Here's how the part is built. I have some questions about the finished solid (model axes, mm). A direction names the side the tool comes from. Round coordinates to 2 decimals unless told otherwise and drop trailing zeros. Order: outer loops, then holes, each group sorted by start corner. A loop starts at its lowest first (then second) coordinate and runs counter-clockwise, first axis right, second up.
```python
from build123d import *

# Parameters (mm, degrees)
SKETCH1_R           = 14.2875
SKETCH1_R_2         = 7.9375
SKETCH1_R_3         = 3.429
SKETCH1_R_4         = 2.54
BOSS_EXTRUDE1_DEPTH = 6.35


with BuildPart() as part:
    # Sketch1 → Boss-Extrude1 (new body)
    with BuildSketch(Plane(origin=(0, 0, 0), x_dir=(0, 0, -1), z_dir=(1, 0, 0))):
        with BuildLine():
            Line((12.7, -88.9), (-1.575652176, -88.9))
            ThreePointArc((-1.575652176, -88.9), (-4.987504689, -87.905535681), (-7.330706623, -85.233625962))
            Line((-7.330706623, -85.233625962), (-16.304501832, -65.989260033))
            ThreePointArc((-16.304501832, -65.989260033), (-19.450268482, -62.883748133), (-23.860481018, -62.583619201))
            ThreePointArc((-23.860481018, -62.583619201), (-35.194449796, -57.475157953), (-31.822423449, -45.509178558))
            ThreePointArc((-31.822423449, -45.509178558), (-29.217505575, -41.937840594), (-29.574405884, -37.53185896))
            Line((-29.574405884, -37.53185896), (-42.070217791, -10.734503848))
            ThreePointArc((-42.070217791, -10.734503848), (-44.064116927, 4.410663713), (-37.010512242, 17.960512242))
            Line((-37.010512242, 17.960512242), (5.544864644, 60.515889128))
            ThreePointArc((5.544864644, 60.515889128), (12.382451565, 63.66408435), (19.411500847, 60.970351952))
            Line((19.411500847, 60.970351952), (75.796601185, 6.873195536))
            ThreePointArc((75.796601185, 6.873195536), (78.685483549, 0.891546289), (76.962077301, -5.523719874))
            Line((76.962077301, -5.523719874), (20.459777301, -84.898719874))
            ThreePointArc((20.459777301, -84.898719874), (17.065328922, -87.840785752), (12.7, -88.9))
        make_face()
        with Locations((-19.05, 0)):
            Circle(SKETCH1_R, mode=Mode.SUBTRACT)
        with Locations((12.7, 38.1)):
            Circle(SKETCH1_R_2, mode=Mode.SUBTRACT)
        with Locations((12.7, -63.5)):
            Circle(SKETCH1_R_2, mode=Mode.SUBTRACT)
        with Locations((-26.561868124, -53.44971901)):
            Circle(SKETCH1_R_3, mode=Mode.SUBTRACT)
        with Locations((12.7, 53.975)):
            Circle(SKETCH1_R_3, mode=Mode.SUBTRACT)
        with Locations((-3.175, -63.5)):
            Circle(SKETCH1_R_3, mode=Mode.SUBTRACT)
        with Locations((12.7, -47.625)):
            Circle(SKETCH1_R_3, mode=Mode.SUBTRACT)
        with Locations((12.7, -79.375)):
            Circle(SKETCH1_R_3, mode=Mode.SUBTRACT)
        with Locations((-3.175, 38.1)):
            Circle(SKETCH1_R_3, mode=Mode.SUBTRACT)
        with Locations((12.7, 22.225)):
            Circle(SKETCH1_R_3, mode=Mode.SUBTRACT)
        with Locations((44.45, 0)):
            Circle(SKETCH1_R, mode=Mode.SUBTRACT)
        with Locations((44.45, 24.7523)):
            Circle(SKETCH1_R_4, mode=Mode.SUBTRACT)
        with Locations((69.2023, 0)):
            Circle(SKETCH1_R_4, mode=Mode.SUBTRACT)
        with Locations((44.45, -24.7523)):
            Circle(SKETCH1_R_4, mode=Mode.SUBTRACT)
        with Locations((19.6977, 0)):
            Circle(SKETCH1_R_4, mode=Mode.SUBTRACT)
    extrude(amount=BOSS_EXTRUDE1_DEPTH)


solid = part.part
```
1. If we section it at B-B, the plane z = -34.5: Write out the boundary of the cut face in (x, y).
Evaluation:
outline: (0, -65.17) - (6.35, -65.17) - (6.35, -10.25) - (0, -10.25) - close; (0, 10.25) - (6.35, 10.25) - (6.35, 46.49) - (0, 46.49) - close
2. If we section it at A-A, the plane y = 0: Write out the boundary of the cut face in (x, z), and give its area (3 significant figures).
Evaluation:
outline: (0, -78.73) - (6.35, -78.73) - (6.35, -71.74) - (0, -71.74) - close; (0, -66.66) - (6.35, -66.66) - (6.35, -58.74) - (0, -58.74) - close; (0, -30.16) - (6.35, -30.16) - (6.35, -22.24) - (0, -22.24) - close; (0, -17.16) - (6.35, -17.16) - (6.35, 4.76) - (0, 4.76) - close; (0, 33.34) - (6.35, 33.34) - (6.35, 44.45) - (0, 44.45) - close
area: 355 mm2
3. On a 3-axis mill with a long thin cutter (end or side, diameter ignored), from which of +Z, -Z, +X, -X, +Y, -Y can I reach the whole of each face in a straight line? I mean faces 1 (the cylindrical face through (3.13, -0.97, -71.55)), 2 (the flat face through (3.131, -24.321, 35.735)). Say none if no direction works.
Evaluation:
face 1: +X, -X
face 2: +Z, +X, -X
4. I'm going to push flat-ended pins straight in: P1, Ø3, axis at x = 2, y = -20.5, coming from the -Z side; P2, Ø1, axis at x = 2.5, y = 48, coming from the -Z side; P3, Ø3, axis at x = 4, y = -29, coming from the -Z side. Where does each tip first touch, or does it pass through?
Evaluation:
P1: stops at z = -67.37
P2: stops at z = -33.45
P3: stops at z = -61.32
5. If we mould it in two halves opening along Z, with no side actions, what happens to faces 3 (the cylindrical face through (3.131, 57.375, -12.254)), 4 (the flat face through (3.131, -44.656, -49.106)), 5 (the cylindrical face through (3.13, 45.97, -11.67)), 6 (the flat face through (0, -12, -18))? For each: released by +Z, released by -Z, zero draft, split by the parting line, or undercut.
Evaluation:
face 3: undercut
face 4: released by -Z
face 5: undercut
face 6: zero draft
6. If we section it at C-C, the plane x = 2.5: State how many separate pieces and enclosed holes the cut face has, and give its area (3 significant figures).
Evaluation:
separate pieces: 1
enclosed holes: 15
area: 9,480 mm2
7. If we section it at D-D, the plane z = -70: Write out the boundary of the cut face in (x, y), and give its area (3 significant figures).
Evaluation:
outline: (0, -15.3) - (6.35, -15.3) - (6.35, -2.41) - (0, -2.41) - close; (0, 2.41) - (6.35, 2.41) - (6.35, 12.43) - (0, 12.43) - close
area: 146 mm2
8. I need wall thicknesses on probe 1 along Y at (x, z) = (4.75, -44.45); probe 2 along Z at (x, y) = (4, 7); probe 3 along Z at (x, y) = (4, 35.5). Which ranges of each line are inside material? Lowest first, please.
Evaluation:
probe 1: y = -51.2 to -27.29, -22.21 to -14.29, 14.29 to 22.21, 27.29 to 36.95
probe 2: z = -75.66 to -56.91, -31.99 to 6.59, 31.51 to 43.47
probe 3: z = -45.96 to -20.2, -5.2 to 0.94, 5.41 to 19.47
